```python
from build123d import *

# Parameters (mm, degrees)
SKIZZE1_W                       = 410
SKIZZE1_H                       = 410
AUFSATZ_LINEAR_AUSTRAGEN1_DEPTH = 5
SKIZZE2_W                       = 97.796702903
SKIZZE2_H                       = 49.6
SCHNITT_LINEAR_AUSTRAGEN1_DEPTH = 5
LINEARES_MUSTER1_COUNT          = 4
LINEARES_MUSTER1_PITCH          = 99.9
SPIEGELN1_COPY_1_SKETCH_W       = 97.796702903
SPIEGELN1_COPY_1_SKETCH_H       = 49.6
SPIEGELN1_COPY_1_DEPTH          = 5
SPIEGELN1_COPY_2_SKETCH_W       = 97.796702903
SPIEGELN1_COPY_2_SKETCH_H       = 49.6
SPIEGELN1_COPY_2_DEPTH          = 5
SPIEGELN1_COPY_3_SKETCH_W       = 97.796702903
SPIEGELN1_COPY_3_SKETCH_H       = 49.6
SPIEGELN1_COPY_3_DEPTH          = 5
SKIZZE3_W                       = 49.6
SKIZZE3_H                       = 41.77912255
SCHNITT_LINEAR_AUSTRAGEN2_DEPTH = 5
LINEARES_MUSTER2_COUNT          = 4
LINEARES_MUSTER2_PITCH          = 99.9
SPIEGELN2_COPY_1_SKETCH_W       = 49.6
SPIEGELN2_COPY_1_SKETCH_H       = 41.77912255
SPIEGELN2_COPY_1_DEPTH          = 5
SPIEGELN2_COPY_2_SKETCH_W       = 49.6
SPIEGELN2_COPY_2_SKETCH_H       = 41.77912255
SPIEGELN2_COPY_2_DEPTH          = 5
SPIEGELN2_COPY_3_SKETCH_W       = 49.6
SPIEGELN2_COPY_3_SKETCH_H       = 41.77912255
SPIEGELN2_COPY_3_DEPTH          = 5
SCHNITT_LINEAR_AUSTRAGEN3_DEPTH = 5
SPIEGELN4_COPY_1_DEPTH          = 5


with BuildPart() as part:
    # Skizze1 → Aufsatz-Linear austragen1 (new body)
    with BuildSketch(Plane.XY):
        with Locations((205, 205)):
            Rectangle(SKIZZE1_W, SKIZZE1_H)
    extrude(amount=AUFSATZ_LINEAR_AUSTRAGEN1_DEPTH)

    # Skizze2 → Schnitt-Linear austragen1 (cut)
    with BuildSketch(Plane.XY.offset(5)):
        with Locations((-43.898351452, 354.85)):
            Rectangle(SKIZZE2_W, SKIZZE2_H)
    schnitt_linear_austragen1 = extrude(amount=-SCHNITT_LINEAR_AUSTRAGEN1_DEPTH, mode=Mode.SUBTRACT)

    # Lineares Muster1: Schnitt-Linear austragen1 ×4
    with Locations(*[(0, -i * LINEARES_MUSTER1_PITCH, 0) for i in range(1, LINEARES_MUSTER1_COUNT)]):
        add(schnitt_linear_austragen1, mode=Mode.SUBTRACT)

    # Spiegeln1: Schnitt-Linear austragen1 across plane
    add(schnitt_linear_austragen1.mirror(Plane(origin=(205, 0, 0), x_dir=(0, 0, 1), z_dir=(1, 0, 0))), mode=Mode.SUBTRACT)

    # Spiegeln1 copy 1 sketch → Spiegeln1 copy 1 (cut)
    with BuildSketch(Plane(origin=(410, -99.9, 5), x_dir=(-1, 0, 0), z_dir=(0, 0, 1))):
        with Locations((-43.898351452, -354.85)):
            Rectangle(SPIEGELN1_COPY_1_SKETCH_W, SPIEGELN1_COPY_1_SKETCH_H)
    extrude(amount=-SPIEGELN1_COPY_1_DEPTH, mode=Mode.SUBTRACT)

    # Spiegeln1 copy 2 sketch → Spiegeln1 copy 2 (cut)
    with BuildSketch(Plane(origin=(410, -199.8, 5), x_dir=(-1, 0, 0), z_dir=(0, 0, 1))):
        with Locations((-43.898351452, -354.85)):
            Rectangle(SPIEGELN1_COPY_2_SKETCH_W, SPIEGELN1_COPY_2_SKETCH_H)
    extrude(amount=-SPIEGELN1_COPY_2_DEPTH, mode=Mode.SUBTRACT)

    # Spiegeln1 copy 3 sketch → Spiegeln1 copy 3 (cut)
    with BuildSketch(Plane(origin=(410, -299.7, 5), x_dir=(-1, 0, 0), z_dir=(0, 0, 1))):
        with Locations((-43.898351452, -354.85)):
            Rectangle(SPIEGELN1_COPY_3_SKETCH_W, SPIEGELN1_COPY_3_SKETCH_H)
    extrude(amount=-SPIEGELN1_COPY_3_DEPTH, mode=Mode.SUBTRACT)

    # Skizze3 → Schnitt-Linear austragen2 (cut)
    with BuildSketch(Plane.XY.offset(5)):
        with Locations((55.15, 425.889561275)):
            Rectangle(SKIZZE3_W, SKIZZE3_H)
    schnitt_linear_austragen2 = extrude(amount=-SCHNITT_LINEAR_AUSTRAGEN2_DEPTH, mode=Mode.SUBTRACT)

    # Lineares Muster2: Schnitt-Linear austragen2 ×4
    with Locations(*[(i * LINEARES_MUSTER2_PITCH, 0, 0) for i in range(1, LINEARES_MUSTER2_COUNT)]):
        add(schnitt_linear_austragen2, mode=Mode.SUBTRACT)

    # Spiegeln2: Schnitt-Linear austragen2 across plane
    add(schnitt_linear_austragen2.mirror(Plane.ZX.offset(205)), mode=Mode.SUBTRACT)

    # Spiegeln2 copy 1 sketch → Spiegeln2 copy 1 (cut)
    with BuildSketch(Plane(origin=(99.9, 410, 5), x_dir=(1, 0, 0), z_dir=(0, 0, 1))):
        with Locations((55.15, -425.889561275)):
            Rectangle(SPIEGELN2_COPY_1_SKETCH_W, SPIEGELN2_COPY_1_SKETCH_H)
    extrude(amount=-SPIEGELN2_COPY_1_DEPTH, mode=Mode.SUBTRACT)

    # Spiegeln2 copy 2 sketch → Spiegeln2 copy 2 (cut)
    with BuildSketch(Plane(origin=(199.8, 410, 5), x_dir=(1, 0, 0), z_dir=(0, 0, 1))):
        with Locations((55.15, -425.889561275)):
            Rectangle(SPIEGELN2_COPY_2_SKETCH_W, SPIEGELN2_COPY_2_SKETCH_H)
    extrude(amount=-SPIEGELN2_COPY_2_DEPTH, mode=Mode.SUBTRACT)

    # Spiegeln2 copy 3 sketch → Spiegeln2 copy 3 (cut)
    with BuildSketch(Plane(origin=(299.7, 410, 5), x_dir=(1, 0, 0), z_dir=(0, 0, 1))):
        with Locations((55.15, -425.889561275)):
            Rectangle(SPIEGELN2_COPY_3_SKETCH_W, SPIEGELN2_COPY_3_SKETCH_H)
    extrude(amount=-SPIEGELN2_COPY_3_DEPTH, mode=Mode.SUBTRACT)

    # Skizze4 → Schnitt-Linear austragen3 (cut)
    with BuildSketch(Plane.XY.offset(5)):
        Polygon((5, 379.65), (5, 405), (30.35, 405), (30.35, 431.549801047), (5, 431.549801047), (-47.862925009, 431.549801047), (-47.862925009, 405), (-47.862925009, 379.65), align=None)
    schnitt_linear_austragen3 = extrude(amount=-SCHNITT_LINEAR_AUSTRAGEN3_DEPTH, mode=Mode.SUBTRACT)

    # Spiegeln3: Schnitt-Linear austragen3 across plane
    add(schnitt_linear_austragen3.mirror(Plane(origin=(205, 0, 0), x_dir=(0, 0, 1), z_dir=(1, 0, 0))), mode=Mode.SUBTRACT)

    # Spiegeln4: Schnitt-Linear austragen3 across plane
    add(schnitt_linear_austragen3.mirror(Plane.ZX.offset(205)), mode=Mode.SUBTRACT)

    # Spiegeln4 copy 1 sketch → Spiegeln4 copy 1 (cut)
    with BuildSketch(Plane(origin=(410, 410, 5), x_dir=(-1, 0, 0), z_dir=(0, 0, 1))):
        Polygon((5, 379.65), (5, 405), (30.35, 405), (30.35, 431.549801047), (5, 431.549801047), (-47.862925009, 431.549801047), (-47.862925009, 405), (-47.862925009, 379.65), align=None)
    extrude(amount=-SPIEGELN4_COPY_1_DEPTH, mode=Mode.SUBTRACT)


solid = part.part
```
The model under review builds one solid part; all positions refer to its coordinate system, in mm. Round coordinates to 2 decimals unless told otherwise and drop trailing zeros. Order: outer loops, then holes, each group sorted by start corner. A loop starts at its lowest first (then second) coordinate and runs counter-clockwise, first axis right, second up. Notation, with made-up numbers: (0.5, 87.25) - (38.5, 87.25) arc R13 cw to (38.5, 104.25) - close; hole circle Ø1 at (-22, -7). An arc over 180 degrees is marked (long way). Answer in a Markdown table with one row per item.
(1) Clearance check with flat-ended pins moving along their axes: P1, Ø2.5, axis at y = 2.5, z = 2, coming from the -X side; P2, Ø1.5, axis at y = 382.5, z = 3.5, coming from the -X side; P3, Ø1.5, axis at x = 408, z = 3.5, coming from the -Y side; P4, Ø4, axis at x = 339.5, y = 159, coming from the -Z side. State where each tip first meets the part, or that it passes through.
Result set:
| item | result |
|---|---|
| P1 | stops at x = 79.95 |
| P2 | stops at x = 5 |
| P3 | stops at y = 79.95 |
| P4 | stops at z = 0 |
(2) For line 1 (Y direction, x = 263, z = 0.5), list the stretches that pass through material, from the lowest coordinate up. Write a range as from..to.
Result set:
| item | result |
|---|---|
| line 1 | y = 5..405 |
(3) Take a section at A-A on x = 153. Write out the cut boundary in (y, z), plus the area to 3 significant figures.
Result set:
| item | result |
|---|---|
| outline | (5, 0) - (405, 0) - (405, 5) - (5, 5) - close |
| area | 2,000 mm2 |
